```python
from build123d import *

# Parameters (mm, degrees)
SKETCH016_W      = 32
SKETCH016_H      = 32
SKETCH016_R      = 9.75
EXTRUDE015_DEPTH = 6
SKETCH017_R      = 10.75
SKETCH017_R_2    = 9.75
EXTRUDE016_DEPTH = 25
SKETCH014_W      = 36
SKETCH014_H      = 36
SKETCH014_W_2    = 28
SKETCH014_H_2    = 28
EXTRUDE013_DEPTH = 2


with BuildPart() as extrude015:
    # Sketch016 → Extrude015 (new body)
    with BuildSketch(Plane.XZ):
        with Locations((-18, -18)):
            Rectangle(SKETCH016_W, SKETCH016_H)
        with Locations((-18, -18)):
            Circle(SKETCH016_R, mode=Mode.SUBTRACT)
    extrude(amount=EXTRUDE015_DEPTH)


with BuildPart() as extrude015_1:
    # Extrude015 placement: moved
    add(extrude015.part.moved(Location((0, -4, 0))))


with BuildPart() as extrude016:
    # Sketch017 → Extrude016 (new body)
    with BuildSketch(Plane.XZ):
        with Locations((-18, -18)):
            Circle(SKETCH017_R)
        with Locations((-18, -18)):
            Circle(SKETCH017_R_2, mode=Mode.SUBTRACT)
    extrude(amount=EXTRUDE016_DEPTH)


with BuildPart() as extrude016_1:
    # Extrude016 placement: moved
    add(extrude016.part.moved(Location((0, -4, 0))))


with BuildPart() as fusion002:
    # Sketch014 → Extrude013 (new body)
    with BuildSketch(Plane.XZ):
        with Locations((-18, -18)):
            Rectangle(SKETCH014_W, SKETCH014_H)
        with Locations((-18, -18)):
            Rectangle(SKETCH014_W_2, SKETCH014_H_2, mode=Mode.SUBTRACT)
    extrude(amount=EXTRUDE013_DEPTH)


with BuildPart() as fusion002_1:
    # Extrude013 placement: moved
    add(fusion002.part.moved(Location((0, -4, 0))))

    # Fusion002: union Extrude015, Extrude016
    add(extrude015_1.part)
    add(extrude016_1.part)


solid = fusion002_1.part
```
Build history of the part. All positions in model axes, mm. A direction names the side the tool comes from. Give positions to 0.01 mm unless a question says otherwise; leave off trailing zeros. Order: outer loops, then holes, each group sorted by start corner. A loop starts at its lowest first (then second) coordinate and runs counter-clockwise, first axis right, second up. Notation, with made-up numbers: M 8,64 L 50,64 A26 cw 50,99 Z; hole C 89,85.5 d2. An arc over 180 degrees is marked long. Write item = value, one per line. Start each with the question number.
(1) Slice it at A-A on x = -18. Write the cut outline in (y, z), plus the area to 3 significant figures.
(2) Slice it at D-D on y = -16. Write the cut outline in (x, z).
(3) Slice it at B-B on z = -18. Write the cut outline in (x, y), plus the area to 3 significant figures.
(4) Slice it at C-C on x = -6. Write the cut outline in (y, z).
(5) Which spindle directions (+Z, -Z, +X, -X, +Y, -Y) get a long thin tool onto all of the face, cutting with end or side? Do faces 5 (the flat face through (-2, -8, -18)), 6 (the flat face through (-18, -10, -7)), 7 (the flat face through (0, -5, -18)), 8 (the flat face through (-34, -8, -18)), 9 (the flat face through (-18, -8, -34)). Say none if no direction does.
(6) Two-plate mould, pull along Z, no slides. Class faces 1 (the cylindrical face through (-7.746, -19.367, -14.771)), 2 (the flat face through (-10, -4, -26)), 3 (the cylindrical face through (-13.5, -16.32, -26.65)), 4 (the flat face through (-18, -8, -2)): released by +Z, released by -Z, zero draft, split by the parting line, or undercut.
(7) Probe L1, parallel to Z at x = -18, y = -20; L2, parallel to Z at x = -18, y = -9; L3, parallel to X at y = -6.75, z = -3. List the from-to ranges inside material, lowest first. Write a range as [from, to].
(8) Pin check, flat tips, straight feed: pin 1 Ø5 at (y, z) = (-23, -23.5) entering from +X; pin 2 Ø3 at (y, z) = (-8.5, -12) entering from -X; pin 3 Ø4 at (y, z) = (-10, -20.5) entering from +X. Stop position of each tip, or through.
Responses:
q1.outline = M -29,-28.75 L -10,-28.75 L -10,-34 L -6,-34 L -6,-36 L -4,-36 L -4,-27.75 L -29,-27.75 Z; M -29,-8.25 L -4,-8.25 L -4,0 L -6,0 L -6,-2 L -10,-2 L -10,-7.25 L -29,-7.25 Z
q1.area = 121 mm2
q2.outline = C -18,-18 d21.5; hole C -18,-18 d19.5
q3.outline = M -36,-6 L -34,-6 L -34,-10 L -28.75,-10 L -28.75,-29 L -27.75,-29 L -27.75,-4 L -36,-4 Z; M -8.25,-29 L -7.25,-29 L -7.25,-10 L -2,-10 L -2,-6 L 0,-6 L 0,-4 L -8.25,-4 Z
q3.area = 121 mm2
q4.outline = M -10,-34 L -6,-34 L -6,-36 L -4,-36 L -4,0 L -6,0 L -6,-2 L -10,-2 Z
q5.face_5 = +Z, -Z, +X, -Y
q5.face_6 = -Y
q5.face_7 = +Z, -Z, +X, +Y, -Y
q5.face_8 = +Z, -Z, -X, -Y
q5.face_9 = -Z, +X, -X, -Y
q6.face_1 = split by the parting line
q6.face_2 = zero draft
q6.face_3 = undercut
q6.face_4 = released by +Z
q7.L1 = [-28.75, -27.75], [-8.25, -7.25]
q7.L2 = [-34, -27.75], [-8.25, -2]
q7.L3 = [-34, -2]
q8.pin_1 = -7.68
q8.pin_2 = -34
q8.pin_3 = -2
